Design review of the part built by this model. Coordinates are the model's own, in mm. Face numbers are marked on the shaded views. A direction names the side the tool comes from. Coordinates: 2 decimals unless noted, no trailing zeros. Loops run counter-clockwise (first coordinate to the right, second up) from the corner with the lowest first, then second, coordinate; pieces in that order, holes last. Notation, with made-up numbers: M 29,50 L 77,50 A21 cw 77,80 Z; hole C 59.5,7.25 d10. An arc over 180 degrees is marked long. Answer as a JSON object with one key per item and string values. Group by question number.
1. To check wall thickness, follow probe 1 along X at (y, z) = (8, 34); probe 2 along Z at (x, y) = (106, 72); probe 3 along Y at (x, z) = (1, 62.5). State the ranges of each line that lie inside material, in increasing order.
2. Insertion check: pin 1 (16 mm diameter, centred on x = 8, z = 6.5, fed in from +Y); pin 2 (16 mm diameter, centred on x = 5.5, z = 180, fed in from +Y). Each pin has a flat end and moves straight along its axis. Give the tip position at first contact, or say it passes through.
3. Consider section D-D (y = 53.5). State the section outline as (x, z) points.
4. Draft analysis for pull direction Z (two halves, no side actions). For the marked faces 1, 2 and 3, state which applies: +Z half, -Z half, draft (parallel to the pull), parting line (faces both ways), or undercut.
5. Consider section A-A (y = 30.5). State the section outline as (x, z) points, then the cut area to 3 significant figures.
6. Machinability: for the marked faces 4 and 5, which of the approach directions +Z, -Z, +X, -X, +Y, -Y give a long, thin tool a straight path to every point of the face, cutting with its end or side? Answer none if there is none.
7. Consider section B-B (x = 9.5). State the section outline as (y, z) points.
8. Consider section C-C (z = 230). State the section outline as (x, y) points.
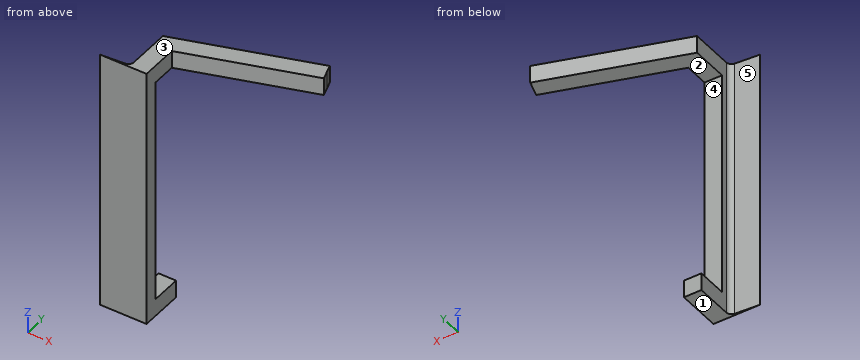
from build123d import *

# Parameters (mm, degrees)
BOSS_EXTRU_2_DEPTH = 300
ESQUISSE7_W        = 20
ESQUISSE7_H        = 20
BOSS_EXTRU_5_DEPTH = 35
BOSS_EXTRU_6_DEPTH = 20


with BuildPart() as part:
    # Esquisse2 → Boss.-Extru.2 (new body)
    with BuildSketch(Plane.XY):
        Polygon((18, 15), (18, 0), (0, 0), (0, 5.028017638), (0, 15), align=None)
        with BuildLine():
            Line((-2, 15), (-2, 7.892441846))
            ThreePointArc((-2, 7.892441846), (-3.612637831, 3.799636794), (-7.583684398, 1.906902495))
            Line((-7.583684398, 1.906902495), (-35, 0))
            Line((-35, 0), (0, 0))
            Line((0, 0), (0, 5.028017638))
            Line((0, 5.028017638), (0, 15))
            Line((0, 15), (-2, 15))
        make_face()
    extrude(amount=BOSS_EXTRU_2_DEPTH)

    # Esquisse7 → Boss.-Extru.5 (add)
    with BuildSketch(Plane(origin=(0, 15, 0), x_dir=(1, 0, 0), z_dir=(0, 1, 0))):
        with Locations((8, -10)):
            Rectangle(ESQUISSE7_W, ESQUISSE7_H)
        with Locations((8, -290)):
            Rectangle(ESQUISSE7_W, ESQUISSE7_H)
    extrude(amount=BOSS_EXTRU_5_DEPTH)

    # Esquisse8 → Boss.-Extru.6 (add)
    with BuildSketch(Plane.XY.offset(300)):
        Polygon((158.049218198, 98.031133425), (155.000575208, 107.555091421), (-2, 57.298811074), (-2, 36.299138452), (161.097861189, 88.507175428), align=None)
    extrude(amount=-BOSS_EXTRU_6_DEPTH)


solid = part.part
Findings below:
{
 "1": {"probe 1": "x = -2 to 18", "probe 2": "z = 280 to 300", "probe 3": "y = 0 to 15"},
 "2": {"pin 1": "stops at y = 50", "pin 2": "stops at y = 15"},
 "3": {"outline": "M -2,280 L 51.74,280 L 51.74,300 L -2,300 Z"},
 "4": {"face 1": "-Z half", "face 2": "undercut", "face 3": "+Z half"},
 "5": {"outline": "M -2,0 L 18,0 L 18,20 L -2,20 Z; M -2,280 L 18,280 L 18,300 L -2,300 Z", "area": "800 mm^2"},
 "6": {"face 4": "+X, -X, +Y", "face 5": "+Z, -Z, -X, +Y"},
 "7": {"outline": "M 0,0 L 50,0 L 50,20 L 15,20 L 15,280 L 60.98,280 L 60.98,300 L 0,300 Z"},
 "8": {"outline": "M -35,0 L 18,0 L 18,15 L -2,15 L -2,7.89 A6 cw -7.58,1.91 Z"}
}
